Source: CAD feature listing. Evaluate the final solid. Frame: model axes, mm. Give positions to 0.01 mm unless a question says otherwise; leave off trailing zeros. Loops run counter-clockwise (first coordinate to the right, second up) from the corner with the lowest first, then second, coordinate; pieces in that order, holes last. Notation, with made-up numbers: (72, 66) - (85, 66) arc R14 ccw to (85, 82) - close; hole circle Ø3 at (26.5, 12). An arc over 180 degrees is marked (long way). Put each result on its own line as item: value.
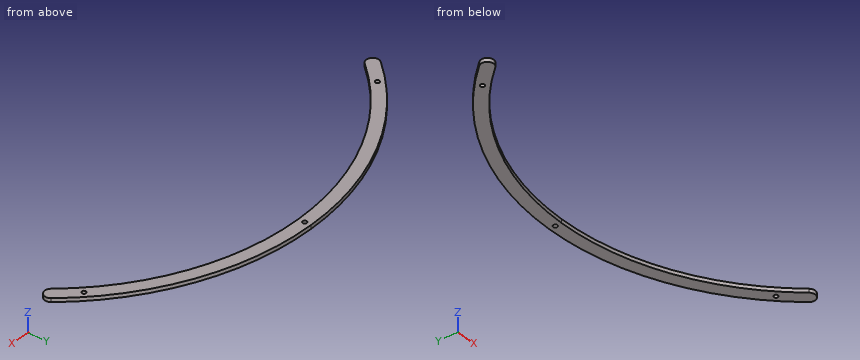
```python
from build123d import *

# Parameters (mm, degrees)
PAD014_DEPTH                        = 3
SKETCH055_R                         = 1.65
POCKET019_DEPTH                     = 364.282338
POCKET019_DEPTH_BACK                = 367.282338
BODY001003005003003_PLACEMENT_ANGLE = 60
CLONE021_PLACEMENT_ANGLE            = 60


with BuildPart() as part:
    # Sketch052 → Pad014 (new body)
    with BuildSketch(Plane.XY):
        with BuildLine():
            ThreePointArc((152.959511, 127.101705), (84.480895, 180.040089), (0, 198.875477))
            Line((0, 198.875477), (0, 208.875477))
            ThreePointArc((160.650731, 133.492724), (88.728824, 189.092995), (0, 208.875477))
            ThreePointArc((152.959511, 127.101705), (160.000631, 126.451604), (160.650731, 133.492724))
        make_face()
    pad014 = extrude(amount=PAD014_DEPTH)

    # Sketch055 → Pocket019 (cut, two sides)
    with BuildSketch(Plane.XY) as pocket019_sk:
        with Locations((143.11, 145.205847)):
            Circle(SKETCH055_R)
        with BuildLine():
            Line((0, 202.225477), (0, 205.525477))
            ThreePointArc((0, 202.225477), (1.65, 203.875477), (0, 205.525477))
        make_face()
    pocket019 = extrude(amount=-POCKET019_DEPTH, mode=Mode.SUBTRACT) + extrude(pocket019_sk.sketch, amount=POCKET019_DEPTH_BACK, mode=Mode.SUBTRACT)

    # Mirrored019: Pad014, Pocket019 across Sketch052 V_Axis
    add(pad014.mirror(Plane(origin=(0, 0, 0), x_dir=(0, 0, 1), z_dir=(1, 0, 0))))
    add(pocket019.mirror(Plane(origin=(0, 0, 0), x_dir=(0, 0, 1), z_dir=(1, 0, 0))), mode=Mode.SUBTRACT)


with BuildPart() as part_1:
    # Body001003005003003 placement: moved
    add(part.part.rotate(Axis((0, 0, 0), (0, 0, 1)), BODY001003005003003_PLACEMENT_ANGLE))


with BuildPart() as part_2:
    # Clone021 placement: moved
    add(part_1.part.moved(Location((0, 62, 0))).rotate(Axis((0, 62, 0), (0, 0, -1)), CLONE021_PLACEMENT_ANGLE))


solid = part_2.part
```
1) Section query B-B, the plane z = 1.5. Output: boundary loops of the cut face in (x, y), plus the area to 3 significant figures.
Check result:
outline: (-160.65, 195.49) arc R5 ccw to (-152.96, 189.1) arc R198.88 cw to (0, 260.88) arc R198.88 cw to (152.96, 189.1) arc R5 ccw to (160.65, 195.49) arc R208.88 ccw to (0, 270.88) arc R208.88 ccw to start; hole circle Ø3.3 at (-143.11, 207.21); hole circle Ø3.3 at (0, 265.88); hole circle Ø3.3 at (143.11, 207.21)
area: 3,630 mm²
2) Pin query (flat end, axial travel): P1, Ø5.5, axis at x = 0, y = 265.88, coming from the -Z side; P2, Ø1.5, axis at x = 123.5, z = 0.5, coming from the +Y side; P3, Ø1, axis at y = 243, z = 1.5, coming from the -X side. Return the tip coordinate at first contact, or that it passes through.
Check result:
P1: z = 0
P2: y = 231
P3: x = -105.11
3) Section query C-C, the plane y = 214.5. Output: boundary loops of the cut face in (x, z).
Check result:
outline: (-142.73, 0) - (-127.65, 0) - (-127.65, 3) - (-142.73, 3) - close; (127.65, 0) - (142.73, 0) - (142.73, 3) - (127.65, 3) - close
4) Material intervals for line 1 along Y through (x, z) = (0, 1.6); line 2 along X through (y, z) = (244, 0.95); line 3 along X through (y, z) = (226, 0.65), sorted ascending. Write a range as [from, to].
Check result:
line 1: [260.88, 264.23], [267.53, 270.88]
line 2: [-102.49, -80.17], [80.17, 102.49]
line 3: [-129.36, -112.5], [112.5, 129.36]
5) Section query A-A, the plane y = 230.5. Output: boundary loops of the cut face in (x, z).
Check result:
outline: (-123.44, 0) - (-105.64, 0) - (-105.64, 3) - (-123.44, 3) - close; (105.64, 0) - (123.44, 0) - (123.44, 3) - (105.64, 3) - close
